Source: CAD feature listing. Evaluate the final solid. Frame: model axes, mm. Face numbers are marked on the shaded views. A direction names the side the tool comes from. Round coordinates to 2 decimals unless told otherwise and drop trailing zeros. Loops run counter-clockwise (first coordinate to the right, second up) from the corner with the lowest first, then second, coordinate; pieces in that order, holes last. Notation, with made-up numbers: M 62.25,63.5 L 88.25,63.5 A5 ccw 88.25,70.5 Z; hole C 72.5,67 d8. An arc over 180 degrees is marked long. One line per item, written item: value.
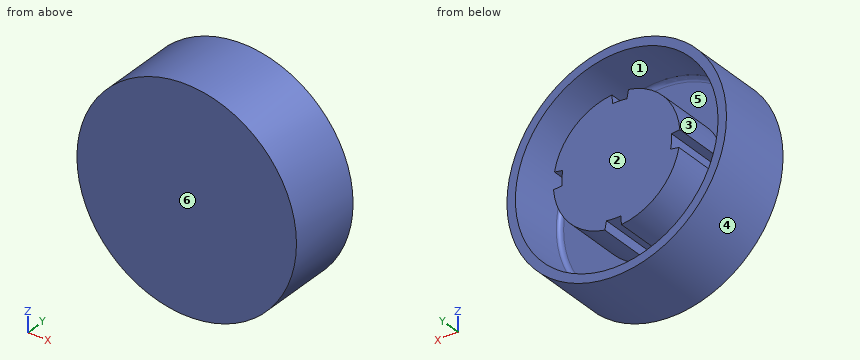
Autodesk Inventor part; units mm, degrees
ref_plane "YZ Plane" through (0, 0, 0) normal (1, 0, 0) x (0, 1, 0)
ref_plane "XZ Plane" through (0, 0, 0) normal (0, 1, 0) x (-1, 0, 0)
ref_plane "XY Plane" through (0, 0, 0) normal (0, 0, 1) x (1, 0, 0)
sketch "Szkic1" plane through (0, 0, 0) normal (0, 1, 0) x (-1, 0, 0)
  circle A0 centre (0, 0) radius 12
  circle A1 centre (0, 0) radius 13
  dimension "d0" = 24
  dimension "d1" = 1
extrude "Wyciągnięcie proste1" add sketch "Szkic1" along normal blind 7
extrude "Wyciągnięcie proste2" add sketch "Szkic1" against normal blind 2 contours A0 | A1
sketch "Szkic2" plane through (0, 0, 0) normal (0, 1, 0) x (1, 0, 0)
  circle A0 centre (0, 0) radius 12
  circle A1 centre (0, 0) radius 1.5
  line L0 (-1.3953, -7.3691) -> (-1.2093, -6.3865)
  arc A2 (-1.2093, -6.3865) -> (0.4849, -6.4819) centre (0, 0) ccw
  line L1 (0.4849, -6.4819) -> (0.5595, -7.4791)
  arc A3 (0.5595, -7.4791) -> (7.3691, -1.3953) centre (0, 0) ccw
  line L2 (7.3691, -1.3953) -> (6.3865, -1.2093)
  arc A4 (6.3865, -1.2093) -> (6.4819, 0.4849) centre (0, 0) ccw
  line L3 (6.4819, 0.4849) -> (7.4791, 0.5595)
  arc A5 (7.4791, 0.5595) -> (1.3953, 7.3691) centre (0, 0) ccw
  line L4 (1.3953, 7.3691) -> (1.2093, 6.3865)
  arc A6 (1.2093, 6.3865) -> (-0.4849, 6.4819) centre (0, 0) ccw
  line L5 (-0.4849, 6.4819) -> (-0.5595, 7.4791)
  arc A7 (-0.5595, 7.4791) -> (-7.3691, 1.3953) centre (0, 0) ccw
  line L6 (-7.3691, 1.3953) -> (-6.3865, 1.2093)
  arc A8 (-6.3865, 1.2093) -> (-6.4819, -0.4849) centre (0, 0) ccw
  line L7 (-6.4819, -0.4849) -> (-7.4791, -0.5595)
  arc A9 (-7.4791, -0.5595) -> (-1.3953, -7.3691) centre (0, 0) ccw
  point P0 (10.4507, -2.3919)
extrude "Wyciągnięcie proste3" add sketch "Szkic2" along normal blind 7 contours A1 | A9 L7 A8 L6 A7 L5 A6 L4 A5 L3 A4 L2 A3 L1 A2 L0
fillet "Zaokrąglenie1" radius 0.5 1 edges at (12, 0, 0)
properties part number "forma"
1. Section query A-A (y = 2). Return the cut outline in (x, z), and give its area (3 significant figures).
Report:
outline: C 0,0 d26; M -7.48,0.56 L -6.48,0.48 A6.5 ccw -6.39,-1.21 L -7.37,-1.4 A7.5 ccw -0.56,-7.48 L -0.48,-6.48 A6.5 ccw 1.21,-6.39 L 1.4,-7.37 A7.5 ccw 7.48,-0.56 L 6.48,-0.48 A6.5 ccw 6.39,1.21 L 7.37,1.4 A7.5 ccw 0.56,7.48 L 0.48,6.48 A6.5 ccw -1.21,6.39 L -1.4,7.37 A7.5 ccw Z; hole C 0,0 d24
area: 248 mm2
2. Pin query (flat end, axial travel): pin 1 (2 mm diameter, centred on y = -0.5, z = 5, fed in from -X); pin 2 (4 mm diameter, centred on y = 1, z = 4, fed in from -X). Return the tip coordinate at first contact, or that it passes through.
Report:
pin 1: stops at x = -12.37
pin 2: stops at x = -12.85
3. Ray query, line 1 (Z direction, x = 0, y = 3); line 2 (X direction, y = 3.75, z = -1). Return the intervals inside material, ascending. Write a range as [from, to].
Report:
line 1: z = [-13, -12], [-6.5, 6.5], [12, 13]
line 2: x = [-12.96, -11.96], [-6.42, 7.43], [11.96, 12.96]
4. Section query B-B (x = 0). Return the cut outline in (y, z).
Report:
outline: M -2,-13 L 7,-13 L 7,-12 L 0.5,-12 A0.5 cw 0,-11.5 L 0,-6.5 L 7,-6.5 L 7,6.5 L 0,6.5 L 0,11.5 A0.5 cw 0.5,12 L 7,12 L 7,13 L -2,13 Z
5. Reachability of the marked faces 1 and 2 from +Z, -Z, +X, -X, +Y, -Y: full face, straight path, thin tool, end or side. Return the list, or none.
Report:
face 1: +Y
face 2: +Z, -Z, +X, -X, +Y
6. Section query C-C (z = 0). Return the cut outline in (x, y), and give its area (3 significant figures).
Report:
outline: M -13,-2 L 13,-2 L 13,7 L 12,7 L 12,0.5 A0.5 cw 11.5,0 L 6.5,0 L 6.5,7 L -6.5,7 L -6.5,0 L -11.5,0 A0.5 cw -12,0.5 L -12,7 L -13,7 Z
area: 157 mm2
7. Pull-direction query (X, two-part tool) for the marked faces 3, 4, 5 and 6; classes: released by +X, released by -X, zero draft, split by the parting line, or undercut.
Report:
face 3: undercut
face 4: split by the parting line
face 5: undercut
face 6: zero draft
8. Section query D-D (y = -1.25). Return the cut outline in (x, z), and give its area (3 significant figures).
Report:
outline: C 0,0 d26
area: 531 mm2
